Input: part model. Units: mm. Frame: model coordinates. Give positions to 0.01 mm unless a question says otherwise; leave off trailing zeros. Order: outer loops, then holes, each group sorted by start corner. A loop starts at its lowest first (then second) coordinate and runs counter-clockwise, first axis right, second up. Notation, with made-up numbers: (80, 31.5) - (122, 31.5) arc R17 ccw to (122, 64.5) - close; hole circle Ø6 at (45, 70). An arc over 180 degrees is marked (long way). Use a Markdown table: item, result.
from build123d import *

# Parameters (mm, degrees)
F1_DEPTH      = 4.9
F1_DEPTH_BACK = 3.9
F2_R          = 4.32
F3_DEPTH      = 8.8
F4_D          = 6.6


with BuildPart() as f5:
    # F0 (on Top) → F5 (revolve)
    with BuildSketch(Plane.XY):
        Polygon((-0.5, 4.99), (0, 4.99), (0.5, 4.99), (4.4, 4.99), (4.4, 6.0935897653), (2.89, 7.61), (0, 7.61), (-2.89, 7.61), (-4.4, 6.0935897653), (-4.4, 4.99), align=None)
        Polygon((0.5, 4.99), (0, 4.99), (-0.5, 4.99), (-0.5, 4.32), (0, 4.32), (0.5, 4.32), align=None)
    revolve(axis=Axis((2.2, 0, 0), (1, 0, 0)))

    # F1 (add, two sides): a face of the model
    f1_faces = [f5.faces().sort_by_distance(p)[0] for p in [
        (-0.5, -4.8488614865, 0),
    ]]
    extrude(f1_faces, amount=-F1_DEPTH)
    extrude(f1_faces, amount=F1_DEPTH_BACK)

    # F2 (on face) → F3 (join, through all)
    with BuildSketch(Plane(origin=(-4.4, 0, 0), x_dir=(0, -1, 0), z_dir=(-1, 0, 0))):
        Circle(F2_R)
    extrude(amount=-F3_DEPTH)

    # F4 (through all)
    with Locations(Plane(origin=(-4.4, 0, 0), x_dir=(0, -1, 0), z_dir=(-1, 0, 0))):
        with Locations((0, 0)):
            Hole(F4_D / 2)


solid = f5.part
1. Pin query (flat end, axial travel): pin 1 (3 mm diameter, centred on x = 1, y = 6, fed in from -Z); pin 2 (1.5 mm diameter, centred on x = -0.5, y = 4.5, fed in from +Z); pin 3 (1.5 mm diameter, centred on x = 1, y = 3.5, fed in from +Z). Return the tip coordinate at first contact, or that it passes through.
Response:
| item | result |
|---|---|
| pin 1 | stops at z = -6.14 |
| pin 2 | stops at z = 6.62 |
| pin 3 | stops at z = 7.1 |
2. Section query C-C (x = 0.5). Return loops of the section in (y, z), then the cut area to 3 significant figures.
Response:
| item | result |
|---|---|
| outline | circle Ø15.22 at (0, 0); hole circle Ø6.6 at (0, 0) |
| area | 148 mm^2 |
3. Mould query, pull axis Z, two halves, no side actions, for faces 1 (the face through (-0.04, -0.991, 7.545)), 2 (the face through (4.4, 3, -3)), 3 (the face through (0.06, -2.43, 2.23)). Classes: pulls with the +Z half, pulls with the -Z half, needs draft (parallel to the pull), parting line crosses it, or undercut.
Response:
| item | result |
|---|---|
| face 1 | parting line crosses it |
| face 2 | needs draft |
| face 3 | undercut |
4. Material intervals for line 1 along Z through (x, y) = (0.25, 0); line 2 along Z through (x, y) = (-3.75, -0.5); line 3 along Y through (x, z) = (3.25, -2.5), sorted ascending.
Response:
| item | result |
|---|---|
| line 1 | z = -7.61 to -3.3, 3.3 to 7.61 |
| line 2 | z = -6.73 to -3.26, 3.26 to 6.73 |
| line 3 | y = -6.8 to -2.15, 2.15 to 6.8 |
5. Section query A-A (y = 0). Return loops of the section in (x, z).
Response:
| item | result |
|---|---|
| outline | (-4.4, -6.09) - (-2.89, -7.61) - (2.89, -7.61) - (4.4, -6.09) - (4.4, -3.3) - (-4.4, -3.3) - close; (-4.4, 3.3) - (4.4, 3.3) - (4.4, 6.09) - (2.89, 7.61) - (-2.89, 7.61) - (-4.4, 6.09) - close |
